The listing builds one solid part. Answer for the finished solid, in the listing's coordinates (mm). A direction names the side the tool comes from. Round coordinates to 2 decimals unless told otherwise and drop trailing zeros. Write each loop counter-clockwise with the first axis right and the second up, starting at its lowest first coordinate (ties: lowest second). Pieces come first, ordered by that corner, then holes. Notation, with made-up numbers: M 83,47 L 96,47 A22 ccw 96,84 Z; hole C 17,74 d11. An arc over 180 degrees is marked long. Answer as CSV lines item,"result". Start each with the question number.
from build123d import *

# Parameters (mm, degrees)
F0_R     = 1.2
F0_R_2   = 1.500002
F0_R_3   = 2.6
F0_R_4   = 3.300001
F1_DEPTH = 2
F2_W     = 1.5
F2_H     = 108.500022
F3_DEPTH = 7
F4_R     = 2
F5_R     = 0.5


# Not quite as in the source:
# - ends of sketch curves that miss each other by under 0.0002 mm in the source are joined


with BuildPart() as f1:
    # F0 (on Front) → F1 (new body)
    with BuildSketch(Plane.XZ):
        Polygon((9.925, 64.250011), (-10.075, 64.250011), (-10.075, -61.250012), (-10.075, -64.250011), (9.925, -64.250011), align=None)
        with BuildLine():
            ThreePointArc((-3.375001, -59.75), (-2.5749995588, -59.549998), (-1.7749982215, -59.7500004152))
            Line((-1.7749982215, -59.7500004152), (-0.875001, -59.75))
            ThreePointArc((-0.875001, -59.75), (-0.275, -61.25), (-0.8750011748, -62.7499988335))
            Line((-0.8750011748, -62.7499988335), (-1.774999, -62.749999))
            ThreePointArc((-1.774999, -62.749999), (-2.5749995588, -62.950001), (-3.375001, -62.749999))
            Line((-3.375001, -62.749999), (-4.274999, -62.749999))
            ThreePointArc((-4.274999, -62.749999), (-4.875, -61.25), (-4.2749988252, -59.7500011665))
            Line((-4.2749988252, -59.7500011665), (-3.375001, -59.75))
        make_face(mode=Mode.SUBTRACT)
        with Locations((-0.074997, -47.24999)):
            Circle(F0_R, mode=Mode.SUBTRACT)
        with BuildLine():
            ThreePointArc((-1.325, -9.14999), (-1.0613958102, -8.5135931898), (-0.424999, -8.249989))
            Line((-0.424999, -8.249989), (0.274999, -8.249989))
            ThreePointArc((0.274999, -8.249989), (0.9113958102, -8.5135931898), (1.175, -9.14999))
            Line((1.175, -9.14999), (1.175, -26.74999))
            Line((1.175, -26.74999), (1.175, -44.34999))
            ThreePointArc((1.175, -44.34999), (0.9113958102, -44.9863868102), (0.274999, -45.249991))
            Line((0.274999, -45.249991), (-0.424999, -45.249991))
            ThreePointArc((-0.424999, -45.249991), (-1.0613958102, -44.9863868102), (-1.325, -44.34999))
            Line((-1.325, -44.34999), (-1.325, -26.74999))
            Line((-1.325, -26.74999), (-1.325, -9.14999))
        make_face(mode=Mode.SUBTRACT)
        with Locations((-0.074997, -6.24999)):
            Circle(F0_R, mode=Mode.SUBTRACT)
        with Locations((-6.125008, 2.249922)):
            Circle(F0_R_2, mode=Mode.SUBTRACT)
        with Locations((-6.125008, 6.499923)):
            Circle(F0_R_2, mode=Mode.SUBTRACT)
        with Locations((-6.125008, 16.249921)):
            Circle(F0_R_2, mode=Mode.SUBTRACT)
        with Locations((-6.125008, 20.249893)):
            Circle(F0_R_2, mode=Mode.SUBTRACT)
        with Locations((-6.125008, 24.499895)):
            Circle(F0_R_2, mode=Mode.SUBTRACT)
        with Locations((-4.125007, 11.74992)):
            Circle(F0_R, mode=Mode.SUBTRACT)
        with Locations((-2.875012, 9.24992)):
            Circle(F0_R, mode=Mode.SUBTRACT)
        with Locations((-1.12501, 3.499919)):
            Circle(F0_R_3, mode=Mode.SUBTRACT)
        with Locations((-1.12501, 14.999919)):
            Circle(F0_R_3, mode=Mode.SUBTRACT)
        with Locations((-4.125007, 29.749892)):
            Circle(F0_R, mode=Mode.SUBTRACT)
        with Locations((-2.875012, 27.249892)):
            Circle(F0_R, mode=Mode.SUBTRACT)
        with Locations((-1.12501, 21.499891)):
            Circle(F0_R_3, mode=Mode.SUBTRACT)
        with Locations((-6.125008, 34.249893)):
            Circle(F0_R_2, mode=Mode.SUBTRACT)
        with Locations((-6.125008, 38.249865)):
            Circle(F0_R_2, mode=Mode.SUBTRACT)
        with Locations((-6.125008, 42.499866)):
            Circle(F0_R_2, mode=Mode.SUBTRACT)
        with Locations((-6.125008, 52.249865)):
            Circle(F0_R_2, mode=Mode.SUBTRACT)
        with Locations((-4.125007, 47.749864)):
            Circle(F0_R, mode=Mode.SUBTRACT)
        with Locations((-2.875012, 45.249864)):
            Circle(F0_R, mode=Mode.SUBTRACT)
        with Locations((-1.12501, 32.999891)):
            Circle(F0_R_3, mode=Mode.SUBTRACT)
        with Locations((-1.12501, 39.499862)):
            Circle(F0_R_3, mode=Mode.SUBTRACT)
        with Locations((-1.12501, 50.999862)):
            Circle(F0_R_3, mode=Mode.SUBTRACT)
        with BuildLine():
            ThreePointArc((-3.3750014152, 62.7500117785), (-2.5749995588, 62.950014), (-1.7749978062, 62.7500113633))
            Line((-1.7749978062, 62.7500113633), (-0.875001, 62.750011))
            ThreePointArc((-0.875001, 62.750011), (-0.275, 61.250012), (-0.8750011748, 59.7500131665))
            Line((-0.8750011748, 59.7500131665), (-1.774999, 59.750012))
            ThreePointArc((-1.774999, 59.750012), (-2.5749995588, 59.55001), (-3.375001, 59.750012))
            Line((-3.375001, 59.750012), (-4.274999, 59.750012))
            ThreePointArc((-4.274999, 59.750012), (-4.875, 61.250012), (-4.2749988252, 62.7500108335))
            Line((-4.2749988252, 62.7500108335), (-3.3750014152, 62.7500117785))
        make_face(mode=Mode.SUBTRACT)
        with Locations((2.374988, 9.249948)):
            Circle(F0_R_4, mode=Mode.SUBTRACT)
        with Locations((4.874988, 3.499919)):
            Circle(F0_R_2, mode=Mode.SUBTRACT)
        with Locations((4.874988, 14.999919)):
            Circle(F0_R_2, mode=Mode.SUBTRACT)
        with Locations((2.374988, 27.24992)):
            Circle(F0_R_4, mode=Mode.SUBTRACT)
        with Locations((4.874988, 21.499891)):
            Circle(F0_R_2, mode=Mode.SUBTRACT)
        with Locations((2.374988, 45.249891)):
            Circle(F0_R_4, mode=Mode.SUBTRACT)
        with Locations((4.874988, 32.999891)):
            Circle(F0_R_2, mode=Mode.SUBTRACT)
        with Locations((4.874988, 39.499862)):
            Circle(F0_R_2, mode=Mode.SUBTRACT)
        with Locations((4.874988, 50.999862)):
            Circle(F0_R_2, mode=Mode.SUBTRACT)
    extrude(amount=F1_DEPTH)

    # F2 (on face) → F3 (join)
    with BuildSketch(Plane.XZ.offset(2)):
        with Locations((-9.325, 0)):
            Rectangle(F2_W, F2_H)
        with Locations((9.175, 0)):
            Rectangle(F2_W, F2_H)
    extrude(amount=-F3_DEPTH)

    # F4
    f4_edges = [f1.edges().sort_by_distance(p)[0] for p in [
        (-9.325, 5, 54.250011),
        (9.175, 5, 54.250011),
        (-9.325, 5, -54.250011),
        (9.175, 5, -54.250011),
    ]]
    fillet(f4_edges, radius=F4_R)

    # F5
    f5_edges = [f1.edges().sort_by_distance(p)[0] for p in [
        (9.175, 0, -54.250011),
        (-9.325, 0, -54.250011),
        (9.175, 0, 54.250011),
        (-9.325, 0, 54.250011),
    ]]
    fillet(f5_edges, radius=F5_R)


solid = f1.part
Q1. The mould has two halves that part along Z. Classify faces 4 (the face through (-9.31, 4.43, -53.65)), 5 (the face through (9.925, 2, -1)), 6 (the face through (-0.34, -0.99, -7.42)): +Z half, -Z half, draft (parallel to the pull), parting line (faces both ways), or undercut.
Q2. Find section B-B (y = 1.75). Determine the outline of the cut face in (x, z) (3 decimals), plus the area to 4 significant figures.
Q3. Each of these flat-tipped pins is pushed along its axis until it touches: P1, Ø1.2, axis at x = 9, y = 1.5, coming from the +Z side; P2, Ø5, axis at x = 4.87, z = 15, coming from the +Y side. Where does it stop, or does it pass through?
Q4. Find section C-C (x = 4.5). Count the separate pieces of the cut face and the enclosed holes in it, plus the area to 3 significant figures.
Q5. Find section A-A (z = -16.5). Determine the outline of the cut face in (x, y) (3 decimals).
Q6. Straight lines are drawn through the part: L1, parallel to Z at x = 1.75, y = -0.5; L2, parallel to X at y = -1, z = 17 (3 decimals); L3, parallel to X at y = 1, z = -32.5 (3 decimals). For each, find the intervals that lie inside material, in ascending order.
Q7. For faces 1 (the face through (-1.325, -1, -27)), 2 (the face through (-8.575, 2, -1)), 3 (the face through (9.19, 4.43, 53.65)), determine the directions among +Z, -Z, +X, -X, +Y, -Y from which every point of the face is accessible in a straight line to the end or side of a thin tool.
Q8. Find section D-D (z = -56). Determine the outline of the cut face in (x, y) (3 decimals).
Reported:
1,face 4,"-Z half"
1,face 5,"draft"
1,face 6,"undercut"
2,outline,"M -10.075,-54.25 L -8.575,-54.25 L -8.575,54.25 L -10.075,54.25 Z; M 8.425,-54.25 L 9.925,-54.25 L 9.925,54.25 L 8.425,54.25 Z"
2,area,"325.5 mm2"
3,P1,"stops at z = 54.25"
3,P2,"stops at y = 0"
4,separate pieces,"10"
4,enclosed holes,"0"
4,area,"192 mm2"
5,outline,"M -10.075,-2 L -1.325,-2 L -1.325,0 L -8.575,0 L -8.575,5 L -10.075,5 Z; M 1.175,-2 L 9.925,-2 L 9.925,5 L 8.425,5 L 8.425,0 L 1.175,0 Z"
6,L1,"z = -64.25 to 6.01, 12.49 to 24.01, 30.49 to 42.01, 48.49 to 64.25"
6,L2,"x = -10.075 to -7.424, -4.826 to -2.786, 0.536 to 9.925"
6,L3,"x = -10.075 to -8.575, 8.425 to 9.925"
7,face 1,"+Y, -Y"
7,face 2,"+Z, -Z, +Y"
7,face 3,"+Z, +X, -X, +Y"
8,outline,"M -10.075,-2 L 9.925,-2 L 9.925,0 L -10.075,0 Z"
